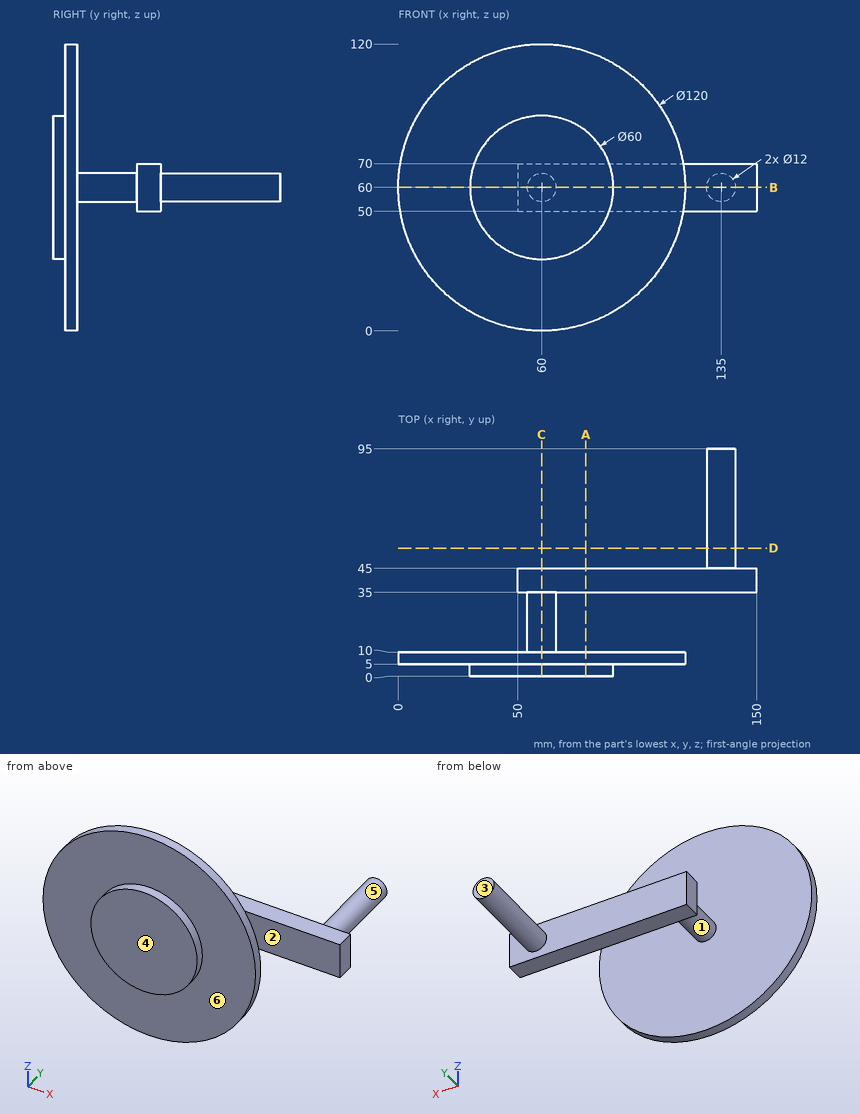
The figure shows three views and two pictorial views of one solid part (mm, origin at its lowest corner). Answer the questions. A direction names the side the tool comes from. Give positions to 0.01 mm unless a question says otherwise; leave off trailing zeros. Loops run counter-clockwise (first coordinate to the right, second up) from the corner with the lowest first, then second, coordinate; pieces in that order, holes last. Notation, with made-up numbers: (-31, 78.5) -> (17, 78.5) arc R27 ccw to (17, 105.5) -> close; hole circle Ø3 at (42, -16.5). An arc over 180 degrees is marked (long way). Put each result on its own line as item: value. Start each with the question number.
Item 1: The part is cut by section A-A (x = 78.5). Give the vertices of the cut face in (y, z), then the cut area to 3 significant figures.
Item 2: The mould has two halves that part along Y. Classify the marked faces 1, 2, 3 and 4: released by +Y, released by -Y, zero draft, split by the parting line, or undercut.
Item 3: Find the intervals of material crossed by L1, parallel to Y at x = 113, z = 61; L2, parallel to X at y = 38, z = 58.5; L3, parallel to Y at x = 45.5, z = 110, in increasing order. Write a range as [from, to].
Item 4: The part is cut by section B-B (z = 60). Give the vertices of the cut face in (x, y).
Item 5: Which of the six approach directions +Z, -Z, +X, -X, +Y, -Y give full straight-line access (tool end or side, diameter ignored) to the marked faces 5 and 6?
Item 6: The part is cut by section D-D (y = 53.5). Give the vertices of the cut face in (x, z).
Item 7: Each of these flat-tipped pins is pushed along its axis until it touches: P1, Ø5, axis at x = 109, y = 42, coming from the -Z side; P2, Ø3, axis at x = 96.5, y = 41, coming from the +Z side; P3, Ø5, axis at x = 79, z = 38, coming from the +Y side; P4, Ø10, axis at x = 117, y = 53, coming from the -Z side. Where does it stop, or does it pass through?
Item 8: The part is cut by section C-C (x = 60). Give the vertices of the cut face in (y, z), then the cut area to 3 significant figures.
Answers below:
1. outline: (0, 36.38) -> (5, 36.38) -> (5, 2.92) -> (10, 2.92) -> (10, 117.08) -> (5, 117.08) -> (5, 83.62) -> (0, 83.62) -> close; (35, 50) -> (45, 50) -> (45, 70) -> (35, 70) -> close
1. area: 1,010 mm2
2. face 1: undercut
2. face 2: undercut
2. face 3: released by +Y
2. face 4: released by -Y
3. L1: [5, 10], [35, 45]
3. L2: [50, 150]
3. L3: [5, 10]
4. outline: (0, 5) -> (30, 5) -> (30, 0) -> (90, 0) -> (90, 5) -> (120, 5) -> (120, 10) -> (66, 10) -> (66, 35) -> (150, 35) -> (150, 45) -> (141, 45) -> (141, 95) -> (129, 95) -> (129, 45) -> (50, 45) -> (50, 35) -> (54, 35) -> (54, 10) -> (0, 10) -> close
5. face 5: +Y
5. face 6: -Y
6. outline: circle Ø12 at (135, 60)
7. P1: z = 50
7. P2: z = 70
7. P3: y = 10
7. P4: through
8. outline: (0, 30) -> (5, 30) -> (5, 0) -> (10, 0) -> (10, 54) -> (35, 54) -> (35, 50) -> (45, 50) -> (45, 70) -> (35, 70) -> (35, 66) -> (10, 66) -> (10, 120) -> (5, 120) -> (5, 90) -> (0, 90) -> close
8. area: 1,400 mm2
